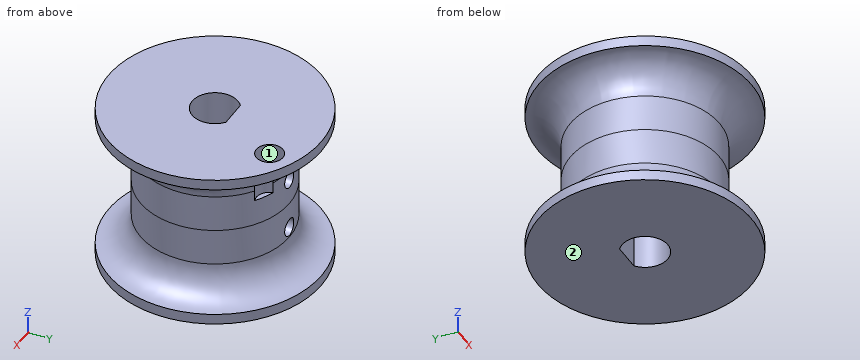
```python
from build123d import *

# Parameters (mm, degrees)
CUT_EXTRUDE1_DEPTH                   = 42.231056256
SKETCH5_W                            = 1.65
SKETCH5_H                            = 20
TAP_DRILL_FOR_M4X0_7_TAP1_AT_2_COUNT = 2
TAP_DRILL_FOR_M4X0_7_TAP1_AT_2_PITCH = 10
FILLET_2_R                           = 6
SKETCH6_R                            = 2.5
CUT_EXTRUDE2_DEPTH                   = 10


with BuildPart() as part:
    # Sketch1 → Revolve1 (revolve)
    with BuildSketch(Plane(origin=(0, 0, 0), x_dir=(0, 0, -1), z_dir=(1, 0, 0))):
        Polygon((0, 0), (0, 14), (13, 14), (13, 20), (15, 20), (15, 0), align=None)
    revolve1 = revolve(axis=Axis((0, 0, -15), (0, 0, 1)))

    # Mirror1: Revolve1 across plane
    add(revolve1.mirror(Plane.XY))

    # Sketch2 → Cut-Extrude1 (cut, through all)
    with BuildSketch(Plane.XY.offset(15)):
        with BuildLine():
            Line((-2.632489316, 3.4), (2.632489316, 3.4))
            ThreePointArc((2.632489316, 3.4), (0, -4.3), (-2.632489316, 3.4))
        make_face()
    extrude(amount=-CUT_EXTRUDE1_DEPTH, mode=Mode.SUBTRACT)

    # Sketch5 → Tap Drill for M4x0.7 Tap1 (revolve, cut)
    with BuildSketch(Plane(origin=(0, 0, -5), x_dir=(0, 0, -1), z_dir=(1, 0, 0))):
        with Locations((0.825, 10)):
            Rectangle(SKETCH5_W, SKETCH5_H)
    tap_drill_for_m4x0_7_tap1 = revolve(axis=Axis((0, -6.35, -5), (0, 1, 0)), mode=Mode.SUBTRACT)

    # Tap Drill for M4x0.7 Tap1 at 2: Tap Drill for M4x0.7 Tap1 ×2
    with Locations(*[(0, 0, i * TAP_DRILL_FOR_M4X0_7_TAP1_AT_2_PITCH) for i in range(1, TAP_DRILL_FOR_M4X0_7_TAP1_AT_2_COUNT)]):
        add(tap_drill_for_m4x0_7_tap1, mode=Mode.SUBTRACT)

    # Fillet 2
    fillet_2_edges = [part.edges().sort_by_distance(p)[0] for p in [
        (0, -14, 13),
        (0, -14, -13),
    ]]
    fillet(fillet_2_edges, radius=FILLET_2_R - 0.0001)  # a hair under: the kernel refuses the full size

    # Sketch6 → Cut-Extrude2 (cut)
    with BuildSketch(Plane.XY.offset(15)):
        with Locations((7, 13.829316686)):
            Circle(SKETCH6_R)
    extrude(amount=-CUT_EXTRUDE2_DEPTH, mode=Mode.SUBTRACT)


solid = part.part
```
Part model, mm, in its own coordinate system. Face numbers are marked on the shaded views. Round coordinates to 2 decimals unless told otherwise and drop trailing zeros. Loops run counter-clockwise (first coordinate to the right, second up) from the corner with the lowest first, then second, coordinate; pieces in that order, holes last.
1. Flat gauge pins, fed straight in: pin 1 (2.5 mm diameter, centred on x = 0, z = 5, fed in from -Y); pin 2 (1.5 mm diameter, centred on y = -9.5, z = -8, fed in from -X); pin 3 (4 mm diameter, centred on y = 3.5, z = -8, fed in from +X). Where does each tip first touch, or does it go through?
Solutions:
pin 1: stops at y = -14
pin 2: stops at x = -11.06
pin 3: stops at x = 14.46
2. Drill centre lines: line 1 along Z through (x, y) = (0, 11.25); line 2 along X through (y, z) = (0, 3); line 3 along Z through (x, y) = (1, 5). Where is each one in solid material? Low to high.
Solutions:
line 1: z = -15 to -6.65, -3.35 to 3.35, 6.65 to 15
line 2: x = -14 to -4.3, 4.3 to 14
line 3: z = -15 to -6.31, -3.69 to 3.69, 6.31 to 15
3. Slice it at C-C (y = 6). Count the separate pieces of the cut face and the enclosed holes in it, and give its area (3 significant figures).
Solutions:
separate pieces: 1
enclosed holes: 2
area: 827 mm2
4. Slice it at D-D (z = -5). Give the cut face in (x, y).
Solutions:
outline: (-2.63, 3.4) - (-1.65, 3.4) - (-1.65, 13.9) arc R14 ccw (long way) to (1.65, 13.9) - (1.65, 3.4) - (2.63, 3.4) arc R4.3 cw (long way) to start
5. Two-plate mould, pull along Y, no slides. Class the marked faces 1 and 2: pulls with the +Y half, pulls with the -Y half, needs draft (parallel to the pull), parting line crosses it, or undercut.
Solutions:
face 1: undercut
face 2: needs draft
6. Slice it at B-B (z = -1). Give the cut face in (x, y), and give its area (3 significant figures).
Solutions:
outline: circle Ø28 at (0, 0); hole (-2.63, 3.4) arc R4.3 ccw (long way) to (2.63, 3.4) - close
area: 561 mm2
